```python
from build123d import *

# Parameters (mm, degrees)
SKETCH_1_W          = 22
SKETCH_1_H          = 17
EXTRUDE_1_DEPTH     = 11
SKETCH_3_W          = 10
SKETCH_3_H          = 17.5
EXTRUDE_2_DEPTH     = 9
SKETCH_4_R          = 1.6
CUT_EXTRUDE_1_DEPTH = 22
SKETCH_5_W          = 8
SKETCH_5_H          = 8
CUT_EXTRUDE_2_DEPTH = 22
FILLET_1_R          = 1.5
FILLET_START        = -6
FILLET_2_DEPTH      = 11
FILLET_START_2      = -5
FILLET_2_2_DEPTH    = 10
SKETCH_7_W          = 37.569031752
SKETCH_7_H          = 53.082934042
CUT_EXTRUDE_4_DEPTH = 22
SKETCH_8_R          = 0.95
EXTRUDE_3_DEPTH     = 1


with BuildPart() as part:
    # 草图1 → 凸台-拉伸1 (new, symmetric)
    with BuildSketch(Plane.XY):
        with Locations((0, -2.5)):
            Rectangle(SKETCH_1_W, SKETCH_1_H)
    extrude(amount=EXTRUDE_1_DEPTH, both=True)

    # 草图2 → 切除-旋转1 (revolve, cut)
    with BuildSketch(Plane.XY, mode=Mode.PRIVATE) as cut_revolve_1_sk:
        with BuildLine():
            Line((0, 6), (6.708203932, 6))
            ThreePointArc((6.708203932, 6), (8.215838363, -3.674234614), (0, -9))
            Line((0, -9), (0, 6))
        make_face()
    revolve(cut_revolve_1_sk.sketch.rotate(Axis((0, 0, 0), (0, 1, 0)), 180), axis=Axis((0, 0, 0), (0, 1, 0)), mode=Mode.SUBTRACT)

    # 草图3 → 凸台-拉伸2 (add, symmetric)
    with BuildSketch(Plane.XY):
        with Locations((0, 14.75)):
            Rectangle(SKETCH_3_W, SKETCH_3_H)
    extrude(amount=EXTRUDE_2_DEPTH, both=True)

    # 草图4 → 切除-拉伸1 (cut)
    with BuildSketch(Plane(origin=(0, 23.5, 0), x_dir=(1, 0, 0), z_dir=(0, 1, 0))):
        with Locations(Location((0, 0, 0), (0, 0, 180))):
            Circle(SKETCH_4_R)
    extrude(amount=-CUT_EXTRUDE_1_DEPTH, mode=Mode.SUBTRACT)

    # 草图5 → 切除-拉伸2 (cut)
    with BuildSketch(Plane.ZY.offset(5)):
        with Locations((0, 10)):
            Rectangle(SKETCH_5_W, SKETCH_5_H)
    extrude(amount=-CUT_EXTRUDE_2_DEPTH, mode=Mode.SUBTRACT)

    # 圆角1
    fillet_1_edges = [part.edges().sort_by_distance(p)[0] for p in [
        (0, -11, 11),
        (11, -2.5, 11),
        (5, 14.75, -9),
        (0, 23.5, -9),
        (5, 23.5, 0),
        (-5, 14.75, -9),
        (-5, 23.5, 0),
        (5, 14.75, 9),
        (0, 23.5, 9),
        (-5, 14.75, 9),
        (0, 6, 11),
        (11, -2.5, -11),
        (0, -11, -11),
        (-11, -2.5, -11),
        (0, 6, -11),
        (11, 6, 0),
        (11, -11, 0),
        (-11, -11, 0),
        (-11, 6, 0),
        (-11, -2.5, 11),
    ]]
    fillet(fillet_1_edges, radius=FILLET_1_R)

    # 圆角2: read off the stored shape, not the designer's step
    # 圆角2 outline → 圆角2 (cut)
    with BuildSketch(Plane.YZ.offset(FILLET_START)):
        with BuildLine():
            Line((6, -4), (6, -5.5))
            ThreePointArc((6, -5.5), (6.439339828, -4.439339828), (7.5, -4))
            Line((7.5, -4), (6, -4))
        make_face()
        with BuildLine():
            Line((6, 4), (7.5, 4))
            ThreePointArc((7.5, 4), (6.439339828, 4.439339828), (6, 5.5))
            Line((6, 5.5), (6, 4))
        make_face()
    extrude(amount=FILLET_2_DEPTH, mode=Mode.SUBTRACT)

    # Fillet 2 2 outline → Fillet 2 2 (add)
    with BuildSketch(Plane.YZ.offset(FILLET_START_2)):
        with BuildLine():
            ThreePointArc((12.5, 4), (13.560660172, 3.560660172), (14, 2.5))
            Line((14, 2.5), (14, 4))
            Line((14, 4), (12.5, 4))
        make_face()
        with BuildLine():
            ThreePointArc((14, -2.5), (13.560660172, -3.560660172), (12.5, -4))
            Line((12.5, -4), (14, -4))
            Line((14, -4), (14, -2.5))
        make_face()
    extrude(amount=FILLET_2_2_DEPTH)

    # 草图7 → 切除-拉伸4 (cut)
    with BuildSketch(Plane(origin=(0, 0, 0), x_dir=(0, 0, -1), z_dir=(1, 0, 0))):
        Rectangle(SKETCH_7_W, SKETCH_7_H)
    extrude(amount=-CUT_EXTRUDE_4_DEPTH, mode=Mode.SUBTRACT)

    # 草图8 → 凸台-拉伸3 (add)
    with BuildSketch(Plane.ZY):
        with Locations(Location((6, 20.5, 0), (0, 0, 180))):
            Circle(SKETCH_8_R)
        with Locations(Location((8.5, -8.5, 0), (0, 0, 180))):
            Circle(SKETCH_8_R)
        with Locations(Location((-6, 20.5, 0), (0, 0, 180))):
            Circle(SKETCH_8_R)
        with Locations(Location((-8.5, -8.5, 0), (0, 0, 180))):
            Circle(SKETCH_8_R)
    extrude(amount=EXTRUDE_3_DEPTH)


solid = part.part
```
Source: CAD feature listing. Evaluate the final solid. Frame: model axes, mm. A direction names the side the tool comes from. Round coordinates to 2 decimals unless told otherwise and drop trailing zeros. Loops run counter-clockwise (first coordinate to the right, second up) from the corner with the lowest first, then second, coordinate; pieces in that order, holes last. Notation, with made-up numbers: M 75,12.5 L 92,12.5 A27 ccw 92,35.5 Z; hole C 73,0.25 d8. An arc over 180 degrees is marked long. Use a Markdown table: item, result. Add a question column.
1. Contact query for flat-ended pins moving along their axis: pin 1 (4 mm diameter, centred on y = 11.5, z = -4, fed in from -X); pin 2 (5 mm diameter, centred on x = 4, y = 6, fed in from +Z); pin 3 (5.5 mm diameter, centred on x = 2, y = 10, fed in from -Z); pin 4 (6 mm diameter, centred on y = 16.5, z = 2, fed in from +X). Output: stop coordinate, or through.
2. Cut plane A-A, the plane y = 11.5. Output: boundary loops of the cut face in (x, z).
3. Set-up query: faces 4 (the cylindrical face through (-0.49, -9.14, 9.2)), 5 (the flat face through (2, 14, 9)), 6 (the cylindrical face through (4.55, 14.11, -8.57)). Return all of +Z, -Z, +X, -X, +Y, -Y with unobstructed straight access to the full face (end or side cutting, diameter ignored); none if empty.
4. Cut plane C-C, the plane x = 6. Output: boundary loops of the cut face in (y, z).
5. Cut plane D-D, the plane y = 20.5. Output: boundary loops of the cut face in (x, z), and give its area (3 significant figures).
6. Pull-direction query (Y, two-part tool) for faces 1 (the cylindrical face through (4.57, 23.05, -0.11)), 2 (the flat face through (3, 14, 0)), 3 (the flat face through (11, -3, 0)); classes: +Y half, -Y half, draft (parallel to the pull), parting line (faces both ways), or undercut.
7. Cut plane B-B, the plane z = 1.25. Output: boundary loops of the cut face in (x, y).
8. Ray query, line 1 along Z through (x, y) = (1, -0.5); line 2 along X through (y, z) = (15.5, 2.25); line 3 along Z through (x, y) = (4, 10). Return the intervals inside material, ascending. Write a range as [from, to].
Solution:
| question | item | result |
|---|---|---|
| 1 | pin 1 | stops at x = 0 |
| 1 | pin 2 | stops at z = 11 |
| 1 | pin 3 | stops at z = -9 |
| 1 | pin 4 | stops at x = 5 |
| 2 | outline | M 0,-9 L 3.5,-9 A1.5 ccw 5,-7.5 L 5,-4 L 0,-4 Z; M 0,4 L 5,4 L 5,7.5 A1.5 ccw 3.5,9 L 0,9 Z |
| 3 | face 4 | -X |
| 3 | face 5 | +Z, +X, -X, +Y |
| 3 | face 6 | -Z, +X, +Y |
| 4 | outline | M -11,-9.5 A1.5 ccw -9.5,-11 L 4.5,-11 A1.5 ccw 6,-9.5 L 6,-3 A6.71 cw long 6,3 L 6,9.5 A1.5 ccw 4.5,11 L -9.5,11 A1.5 ccw -11,9.5 Z |
| 5 | outline | M -1,-6.95 L 0,-6.95 L 0,-9 L 3.5,-9 A1.5 ccw 5,-7.5 L 5,7.5 A1.5 ccw 3.5,9 L 0,9 L 0,6.95 L -1,6.95 L -1,5.05 L 0,5.05 L 0,1.6 A1.6 cw 0,-1.6 L 0,-5.05 L -1,-5.05 Z |
| 5 | area | 88.8 mm2 |
| 6 | face 1 | +Y half |
| 6 | face 2 | undercut |
| 6 | face 3 | draft |
| 7 | outline | M 0,-11 L 9.5,-11 A1.5 ccw 11,-9.5 L 11,4.5 A1.5 ccw 9.5,6 L 6.59,6 A8.91 cw 0,-8.91 Z; M 1,14 L 5,14 L 5,22 A1.5 ccw 3.5,23.5 L 1,23.5 Z |
| 8 | line 1 | z = [-11, -8.93], [8.93, 11] |
| 8 | line 2 | x = [0, 5] |
| 8 | line 3 | z = [-8.91, -4], [4, 8.91] |
